```python
from build123d import *

# Parameters (mm, degrees)
ESBO_O1_R                = 1.5
ESBO_O1_W                = 23
ESBO_O1_H                = 12.5
RESSALTO_EXTRUS_O1_DEPTH = 3


with BuildPart() as part:
    # Esboço1 → Ressalto-extrusão1 (new body)
    with BuildSketch(Plane.XY):
        Polygon((11.242500706, -13), (11.242500706, -8), (12.617500706, -8), (12.617500706, -5.5), (11.242500706, -5.5), (11.242500706, 0), (8.242500706, 0), (8.242500706, -5.5), (6.867500706, -5.5), (6.867500706, -8), (8.242500706, -8), (8.242500706, -13), (-14.857499294, -13), (-14.857499294, -16), (-22.857499294, -16), (-22.857499294, -13), (-22.857499294, 25.3), (-22.857499294, 47), (-20.357499294, 47), (-20.357499294, 42), (-21.732499294, 42), (-21.732499294, 39.5), (-20.357499294, 39.5), (-20.357499294, 34), (-17.357499294, 34), (-17.357499294, 39.5), (-15.982499294, 39.5), (-15.982499294, 42), (-17.357499294, 42), (-17.357499294, 47), (5.742500706, 47), (5.742500706, 50), (13.742500706, 50), (13.742500706, -13), align=None)
        with Locations((-18.857499294, 17)):
            Circle(ESBO_O1_R, mode=Mode.SUBTRACT)
        with Locations((9.742500706, 17)):
            Circle(ESBO_O1_R, mode=Mode.SUBTRACT)
        with Locations((-4.557499294, 17)):
            Rectangle(ESBO_O1_W, ESBO_O1_H, mode=Mode.SUBTRACT)
    extrude(amount=RESSALTO_EXTRUS_O1_DEPTH)


solid = part.part
```
Verification items for the finished model (mm, model axes). A direction names the side the tool comes from. Give positions to 0.01 mm unless a question says otherwise; leave off trailing zeros. Loops run counter-clockwise (first coordinate to the right, second up) from the corner with the lowest first, then second, coordinate; pieces in that order, holes last.
1. Section check D-D, the plane z = 1.65. Count the separate pieces of the cut face and the enclosed holes in it, then the cut area to 3 significant figures.
2. Set-up check for faces 5 (the flat face through (-17.357, 44, 1)), 6 (the flat face through (-17, 42, 1)), 7 (the flat face through (8.243, -3, 1)): record each of +Z, -Z, +X, -X, +Y, -Y from which the full face is reachable in a straight line by a thin tool's end or side.
3. Section check C-C, the plane y = 17. Enter the section's corners in (x, z), then the cut area to 3 significant figures.
4. Go/stop test with flat-tipped pins: pin 1 Ø1.5 at (x, z) = (-4, 1.5) entering from -Y; pin 2 Ø1.5 at (x, z) = (-5, 1.5) entering from +Y; pin 3 Ø1.5 at (x, z) = (9.5, 1.5) entering from -Y. Record where each tip stops, or that it passes through.
5. Section check B-B, the plane y = -3.5. Enter the section's corners in (x, z).
6. Mould release check, pull along X, two halves, no side actions. Record for faces 1 (the flat face through (11.243, -3, 1)), 2 (the flat face through (-14.857, -14, 1)), 3 (the flat face through (-22.857, 16, 1)), 4 (the flat face through (10, 50, 1)): released by +X, released by -X, zero draft, split by the parting line, or undercut.
7. Section check A-A, the plane x = -8. Enter the section's corners in (y, z).
8. Thickness scan on line 1 (Y direction, x = 8, z = 0.9); line 2 (X direction, y = 39, z = 2); line 3 (Y direction, x = -5, z = 0.2). Record the ranges inside material, lowest first.
Geometry says:
1. separate pieces: 1
1. enclosed holes: 3
1. area: 1,850 mm2
2. face 5: +Z, -Z, +Y
2. face 6: +Z, -Z
2. face 7: +Z, -Z, -Y
3. outline: (-22.86, 0) - (-20.36, 0) - (-20.36, 3) - (-22.86, 3) - close; (-17.36, 0) - (-16.06, 0) - (-16.06, 3) - (-17.36, 3) - close; (6.94, 0) - (8.24, 0) - (8.24, 3) - (6.94, 3) - close; (11.24, 0) - (13.74, 0) - (13.74, 3) - (11.24, 3) - close
3. area: 22.8 mm2
4. pin 1: stops at y = -13
4. pin 2: stops at y = 47
4. pin 3: stops at y = 0
5. outline: (-22.86, 0) - (8.24, 0) - (8.24, 3) - (-22.86, 3) - close; (11.24, 0) - (13.74, 0) - (13.74, 3) - (11.24, 3) - close
6. face 1: undercut
6. face 2: released by +X
6. face 3: released by -X
6. face 4: zero draft
7. outline: (-13, 0) - (10.75, 0) - (10.75, 3) - (-13, 3) - close; (23.25, 0) - (47, 0) - (47, 3) - (23.25, 3) - close
8. line 1: y = -13 to -8, -5.5 to 50
8. line 2: x = -22.86 to -20.36, -17.36 to 13.74
8. line 3: y = -13 to 10.75, 23.25 to 47
